from build123d import *

# Parameters (mm, degrees)
SKETCH1_W               = 38
SKETCH1_H               = 9.5
BOSS_EXTRUDE1_DEPTH     = 2.5
SKETCH2_W               = 1.5
SKETCH2_H               = 0.3
CUT_EXTRUDE1_DEPTH      = 2
LPATTERN1_COUNT         = 14
LPATTERN1_PITCH         = 2.7
LPATTERN1_COUNT_DIR2    = 2
LPATTERN1_PITCH_DIR2    = 8.8
CUT_EXTRUDE2_DEPTH      = 1
CUT_EXTRUDE2_DEPTH_BACK = 39
CUT_EXTRUDE3_DEPTH      = 2.5


with BuildPart() as part:
    # Sketch1 → Boss-Extrude1 (new body)
    with BuildSketch(Plane(origin=(0, 0, 0), x_dir=(1, 0, 0), z_dir=(0, 1, 0))):
        with Locations((19, 4.75)):
            Rectangle(SKETCH1_W, SKETCH1_H)
    extrude(amount=BOSS_EXTRUDE1_DEPTH)

    # Sketch2 → Cut-Extrude1 (cut)
    with BuildSketch(Plane(origin=(0, 2.5, 0), x_dir=(1, 0, 0), z_dir=(0, 1, 0))):
        with Locations((1.25, 0.35)):
            Rectangle(SKETCH2_W, SKETCH2_H)
    cut_extrude1 = extrude(amount=-CUT_EXTRUDE1_DEPTH, mode=Mode.SUBTRACT)

    # LPattern1: Cut-Extrude1 14 × 2
    with Locations(*[(i * LPATTERN1_PITCH, 0, -j * LPATTERN1_PITCH_DIR2) for i in range(LPATTERN1_COUNT) for j in range(LPATTERN1_COUNT_DIR2) if (i, j) != (0, 0)]):
        add(cut_extrude1, mode=Mode.SUBTRACT)

    # Sketch4 → Cut-Extrude2 (cut, two sides)
    with BuildSketch(Plane(origin=(38, 0, 0), x_dir=(0, 0, -1), z_dir=(1, 0, 0))) as cut_extrude2_sk:
        Polygon((0.75, 30.700274723), (0.75, 2.5), (0.75, 2.07179677), (4.75, 1), (8.75, 2.07179677), (8.75, 2.5), (8.75, 30.700274723), (8.75, 87.10082417), (0.75, 87.10082417), align=None)
    extrude(amount=CUT_EXTRUDE2_DEPTH, mode=Mode.SUBTRACT)
    extrude(cut_extrude2_sk.sketch, amount=-CUT_EXTRUDE2_DEPTH_BACK, mode=Mode.SUBTRACT)

    # Sketch5 → Cut-Extrude3 (cut)
    with BuildSketch(Plane.ZY):
        Polygon((-0.75, 2.5), (-0.75, 2.07179677), (-4.75, 1), (-8.75, 2.07179677), (-8.75, 2.5), (-9.5, 2.5), (-9.5, 0), (0, 0), (0, 2.5), align=None)
    extrude(amount=-CUT_EXTRUDE3_DEPTH, mode=Mode.SUBTRACT)


solid = part.part
Build history of the part. All positions in model axes, mm. Round coordinates to 2 decimals unless told otherwise and drop trailing zeros. Loops run counter-clockwise (first coordinate to the right, second up) from the corner with the lowest first, then second, coordinate; pieces in that order, holes last. Notation, with made-up numbers: (64, -5.5) -> (110, -5.5) arc R5 ccw to (110, -0.5) -> close; hole circle Ø9 at (18, 5). An arc over 180 degrees is marked (long way). Use CSV: the item, a comma, the result in double quotes. Start each with the question number.
Q1. Flat gauge pin, fed straight in: pin 1 Ø2 at (x, z) = (24, -3.5) entering from +Y. Where does the tip first touch, or does it go through?
Q2. Saw through at A-A on x = 10.5. Give the cut face in (y, z), and give its area (3 significant figures).
Q3. Mould opens along X. For faces 1 (the face through (20, 1, 0)), 2 (the face through (15, 2, -9)) say: +X half, -X half, draft (parallel to the pull), parting line (faces both ways), or undercut.
Q4. Saw through at C-C on x = 28.5. Give the cut face in (y, z).
Q5. Drill centre lines: L1, parallel to Z at x = 15, y = 0.6; L2, parallel to Z at x = 23, y = 2.4; L3, parallel to Y at x = 7.5, z = -4.75. Where is each one in solid material? Low to high.
Q6. Saw through at B-B on y = 1.5. Count the separate pieces of the cut face and the enclosed holes in it, and give its area (3 significant figures).
Q7. Saw through at D-D on z = -3.5. Give the cut face in (x, y), and give its area (3 significant figures).
Solutions:
1,pin 1,"stops at y = 1.6"
2,outline,"(0, -9.5) -> (2.5, -9.5) -> (2.5, -8.75) -> (2.07, -8.75) -> (1, -4.75) -> (2.07, -0.75) -> (2.5, -0.75) -> (2.5, 0) -> (0, 0) -> close"
2,area,"16.0 mm^2"
3,face 1,"draft"
3,face 2,"undercut"
4,outline,"(0, -9.5) -> (2.5, -9.5) -> (2.5, -9.3) -> (0.5, -9.3) -> (0.5, -9) -> (2.5, -9) -> (2.5, -8.75) -> (2.07, -8.75) -> (1, -4.75) -> (2.07, -0.75) -> (2.5, -0.75) -> (2.5, -0.5) -> (0.5, -0.5) -> (0.5, -0.2) -> (2.5, -0.2) -> (2.5, 0) -> (0, 0) -> close"
5,L1,"z = -9.5 to -9.3, -9 to -0.5, -0.2 to 0"
5,L2,"z = -9.5 to -9.3, -9 to -8.75, -0.75 to -0.5, -0.2 to 0"
5,L3,"y = 0 to 1"
6,separate pieces,"2"
6,enclosed holes,"26"
6,area,"193 mm^2"
7,outline,"(2.5, 0) -> (38, 0) -> (38, 1.33) -> (2.5, 1.33) -> close"
7,area,"47.4 mm^2"
